Here's how the part is built. I have some questions about the finished solid (model axes, mm). A direction names the side the tool comes from. Round coordinates to 2 decimals unless told otherwise and drop trailing zeros. Order: outer loops, then holes, each group sorted by start corner. A loop starts at its lowest first (then second) coordinate and runs counter-clockwise, first axis right, second up. Notation, with made-up numbers: (38.25, -14.5) -> (68.25, -14.5) arc R28 ccw to (68.25, 24.5) -> close; hole circle Ø5 at (86.25, 40). An arc over 180 degrees is marked (long way). Use a Markdown table: item, result. Add a question column.
(1) I want a section at C-C, the plane x = 30.5. Please give me the cut outline in (y, z) (1 decimal).
(2) On a 3-axis mill with a long thin cutter (end or side, diameter ignored), from which of +Z, -Z, +X, -X, +Y, -Y can I reach the whole of each face in a straight line? I mean faces 5 (the face through (-1.76, -41.48, -92.16)), 6 (the face through (3.175, -3, -89)), 7 (the face through (-38, -6.35, -51)). Say none if no direction works.
(3) If I drill on probe 1 along Y at (x, z) = (0, -8.95); probe 2 along X at (y, z) = (-5.5, -87) (3 decimals); probe 3 along Y at (x, z) = (42.5, -35.5), over which ranges is the centre line in solid material (lowest first)?
(4) Thinking about a two-plate mould opening in X: for faces 1 (the face through (38, -50.8, -64)), 2 (the face through (-15.259, -12.878, -2.346)), 3 (the face through (0, -6.35, -89)), 4 (the face through (3.175, -3, -13)), which applies, pulls with the +X half, pulls with the -X half, needs draft (parallel to the pull), parting line crosses it, or undercut?
(5) I want a section at D-D, the plane y = -46. Please give me the cut outline in (x, z) (1 decimal), then the cut area to 3 significant figures.
(6) I'm going to push flat-ended pins straight in: P1, Ø1.9, axis at y = -2, z = -52.5, coming from the -X side; P2, Ø2, axis at x = 38, z = -52, coming from the -Y side; P3, Ø6, axis at x = -32, y = -12, coming from the +Z side; P4, Ø7, axis at x = 0, y = -38.1, coming from the -Z side. Where does each tip first touch, or does it pass through?
(7) I want a section at B-B, the plane y = -38.1. Please give me the cut outline in (x, z) (1 decimal).
from build123d import *

# Parameters (mm, degrees)
SKETCH8_R           = 3.81
CUT_EXTRUDE2_DEPTH  = 10.16
CIRPATTERN1_COUNT   = 6
SKETCH10_R          = 40.005
CUT_EXTRUDE4_DEPTH  = 51.8000001
SKETCH16_R          = 5.079288484
BOSS_EXTRUDE1_DEPTH = 10.16
SKETCH17_W          = 6.35
SKETCH17_H          = 6.35
BOSS_EXTRUDE2_DEPTH = 4.7625
CIRPATTERN2_COUNT   = 4


with BuildPart() as part:
    # Sketch1 → Revolve1 (revolve)
    with BuildSketch(Plane(origin=(0, 0, 0), x_dir=(0, 0, -1), z_dir=(1, 0, 0))):
        Polygon((0, 0), (0, -25.4), (7.9375, -25.4), (7.9375, -50.8), (12.7, -50.8), (12.7, 0), align=None)
    revolve(axis=Axis((0, 24.668312757, -50.8), (0, -1, 0)))

    # Sketch8 → Cut-Extrude2 (cut, symmetric)
    with BuildSketch(Plane.XY.offset(-8.282540139)):
        with Locations((0, -38.1)):
            Circle(SKETCH8_R)
    cut_extrude2 = extrude(amount=CUT_EXTRUDE2_DEPTH, both=True, mode=Mode.SUBTRACT)

    # CirPattern1: Cut-Extrude2 ×6 about axis
    cirpattern1_axis = Axis((0, 24.668312757, -50.8), (0, 1, 0))
    for i in range(1, CIRPATTERN1_COUNT):
        add(cut_extrude2.rotate(cirpattern1_axis, i * 360 / CIRPATTERN1_COUNT), mode=Mode.SUBTRACT)

    # Sketch10 → Cut-Extrude4 (cut, through all)
    with BuildSketch(Plane.XZ.offset(50.8)):
        with Locations((0, -50.8)):
            Circle(SKETCH10_R)
    extrude(amount=-CUT_EXTRUDE4_DEPTH, mode=Mode.SUBTRACT)

    # Sketch16 → Boss-Extrude1 (add)
    with BuildSketch(Plane(origin=(0, 0, 0), x_dir=(1, 0, 0), z_dir=(0, 1, 0))):
        with Locations((4.452646476, 5.350182374)):
            Circle(SKETCH16_R)
    extrude(amount=BOSS_EXTRUDE1_DEPTH)

    # Sketch17 → Boss-Extrude2 (add)
    with BuildSketch(Plane.XY.offset(-10.16)):
        with Locations((0, -3.175)):
            Rectangle(SKETCH17_W, SKETCH17_H)
    boss_extrude2 = extrude(amount=-BOSS_EXTRUDE2_DEPTH)

    # CirPattern2: Boss-Extrude2 ×4 about axis
    cirpattern2_axis = Axis((0, 0, -50.8), (0, 1, 0))
    for i in range(1, CIRPATTERN2_COUNT):
        add(boss_extrude2.rotate(cirpattern2_axis, i * 360 / CIRPATTERN2_COUNT))


solid = part.part
Taken from the geometry:
| question | item | result |
|---|---|---|
| 1 | outline | (-50.8, -80.9) -> (-25.4, -80.9) -> (-25.4, -91.4) -> (0, -91.4) -> (0, -76.7) -> (-50.8, -76.7) -> close; (-50.8, -24.9) -> (0, -24.9) -> (0, -10.2) -> (-25.4, -10.2) -> (-25.4, -20.7) -> (-50.8, -20.7) -> close |
| 2 | face 5 | +Z, -Z |
| 2 | face 6 | +Y, -Y |
| 2 | face 7 | -Y |
| 3 | probe 1 | y = -50.8 to -41.91, -34.29 to 0 |
| 3 | probe 2 | x = -35.64 to -17.028, -3.175 to 3.175, 17.028 to 35.64 |
| 3 | probe 3 | y = -25.4 to 0 |
| 4 | face 1 | needs draft |
| 4 | face 2 | parting line crosses it |
| 4 | face 3 | undercut |
| 4 | face 4 | undercut |
| 5 | outline | circle Ø85.7 at (0, -50.8); hole circle Ø80 at (0, -50.8) |
| 5 | area | 744 mm2 |
| 6 | P1 | stops at x = -50.79 |
| 6 | P2 | stops at y = -6.35 |
| 6 | P3 | stops at z = -9.09 |
| 6 | P4 | passes through |
| 7 | outline | (-38.9, -68.8) -> (-36.4, -67.4) arc R40 cw to (-36.4, -34.2) -> (-38.9, -32.8) arc R42.9 ccw to start; (-35.1, -75.4) arc R42.9 ccw to (-3.8, -93.5) -> (-3.8, -90.6) arc R40 cw to (-32.6, -74) -> close; (-35.1, -26.2) -> (-32.6, -27.6) arc R40 cw to (-3.8, -11) -> (-3.8, -8.1) arc R42.9 ccw to start; (3.8, -93.5) arc R42.9 ccw to (35.1, -75.4) -> (32.6, -74) arc R40 cw to (3.8, -90.6) -> close; (3.8, -11) arc R40 cw to (32.6, -27.6) -> (35.1, -26.2) arc R42.9 ccw to (3.8, -8.1) -> close; (36.4, -67.4) -> (38.9, -68.8) arc R42.9 ccw to (38.9, -32.8) -> (36.4, -34.2) arc R40 cw to start |
